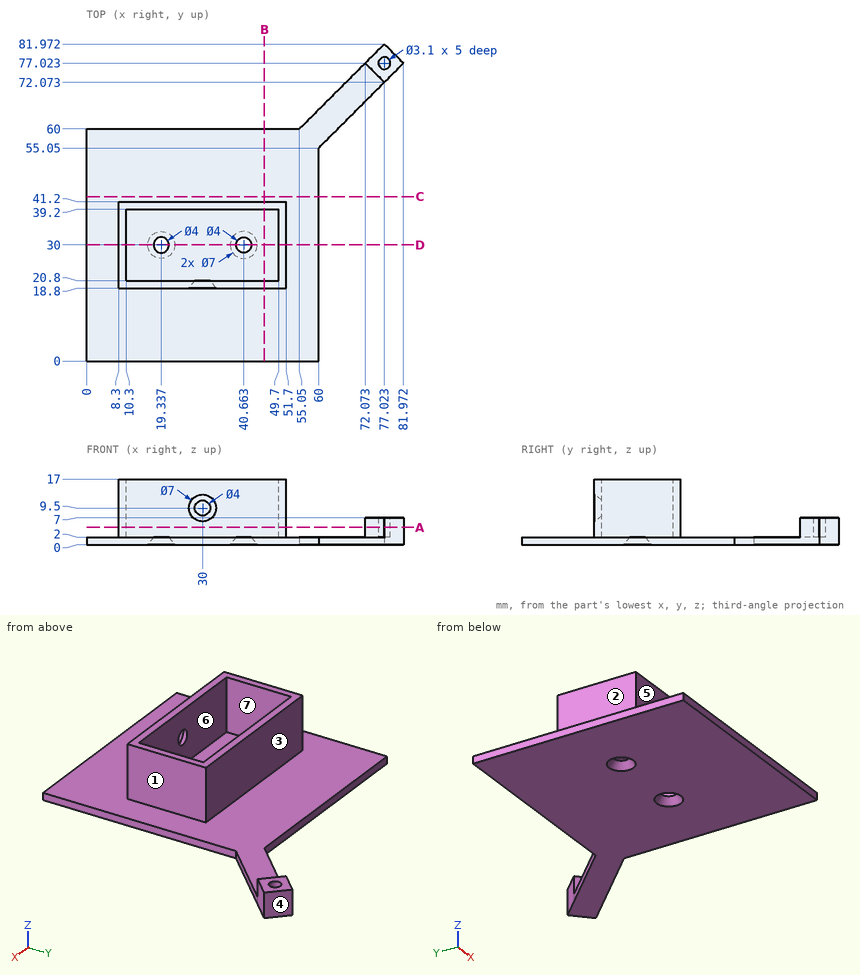
Can you work these out from the drawing? Everything is in mm from the part's minimum corner. A direction names the side the tool comes from. Give positions to 0.01 mm unless a question says otherwise; leave off trailing zeros. Order: outer loops, then holes, each group sorted by start corner. A loop starts at its lowest first (then second) coordinate and runs counter-clockwise, first axis right, second up. Notation, with made-up numbers: (44.25, -30.75) -> (103.25, -30.75) arc R17 ccw to (103.25, -6.75) -> close; hole circle Ø3 at (35.5, 76.5). An arc over 180 degrees is marked (long way). Return JSON: item names as keys, results as strings.
1. On a 3-axis mill with a long thin cutter (end or side, diameter ignored), from which of +Z, -Z, +X, -X, +Y, -Y can I reach the whole of each face in a straight line? I mean the marked faces 1, 2 and 3. Say none if no direction works.
Answer list:
{"face 1": "+Z, +X, +Y, -Y", "face 2": "+Z, -X, +Y, -Y", "face 3": "+Z, +X, -X, +Y"}
2. Imagine slicing it at D-D on y = 30. Give the number of separate pieces and of enclosed holes in the cut face, then the cut area to 3 significant figures.
Answer list:
{"separate pieces": "3", "enclosed holes": "0", "area": "158 mm2"}
3. Imagine slicing it at C-C on y = 42.5. List the corners of the cut face in (x, z) for me, then the cut area to 3 significant figures.
Answer list:
{"outline": "(0, 0) -> (60, 0) -> (60, 2) -> (0, 2) -> close", "area": "120 mm2"}
4. Thinking about a two-plate mould opening in Y: for the marked faces 4, 5, 6 and 7, which applies, pulls with the +Y half, pulls with the -Y half, needs draft (parallel to the pull), parting line crosses it, or undercut?
Answer list:
{"face 4": "pulls with the +Y half", "face 5": "pulls with the -Y half", "face 6": "undercut", "face 7": "undercut"}
5. Imagine slicing it at A-A on z = 4.5. List the corners of the cut face in (x, y) for me.
Answer list:
{"outline": "(8.3, 18.8) -> (51.7, 18.8) -> (51.7, 41.2) -> (8.3, 41.2) -> close; (72.07, 77.02) -> (77.02, 72.07) -> (81.97, 77.02) -> (77.02, 81.97) -> close; hole (10.3, 20.8) -> (49.7, 20.8) -> (49.7, 39.2) -> (10.3, 39.2) -> close; hole circle Ø3.1 at (77.02, 77.02)"}
6. I need wall thicknesses on line 1 (Y direction, x = 26.5, z = 15); line 2 (X direction, y = 37.5, z = 12.5); line 3 (X direction, y = 40, z = 14.5). Which ranges of each line are inside material? Lowest first, please. Write a range as from..to.
Answer list:
{"line 1": "y = 18.8..20.8, 39.2..41.2", "line 2": "x = 8.3..10.3, 49.7..51.7", "line 3": "x = 8.3..51.7"}
7. Imagine slicing it at B-B on x = 46. List the corners of the cut face in (y, z) for me, then the cut area to 3 significant figures.
Answer list:
{"outline": "(0, 0) -> (60, 0) -> (60, 2) -> (41.2, 2) -> (41.2, 17) -> (39.2, 17) -> (39.2, 2) -> (20.8, 2) -> (20.8, 17) -> (18.8, 17) -> (18.8, 2) -> (0, 2) -> close", "area": "180 mm2"}
8. For pin 1 Ø8 at (x, y) = (75.5, 76) entering from +Z; pin 2 Ø4 at (x, y) = (63.5, 27.5) entering from -Z (3 decimals); pin 3 Ø4.5 at (x, z) = (37.5, 12.5) entering from +Y; pin 4 Ø2 at (x, z) = (17, 1.5) entering from +Y, each with a flat end and sliding along its axis, tell me the tip position at first contact or that it passes through.
Answer list:
{"pin 1": "stops at z = 7", "pin 2": "passes through", "pin 3": "stops at y = 41.2", "pin 4": "stops at y = 60"}
